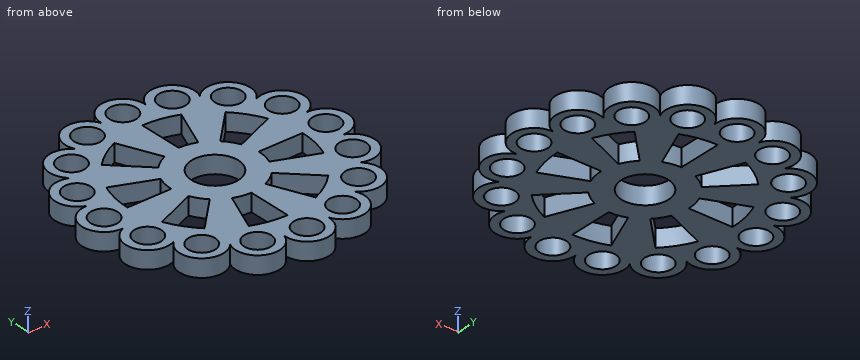
from build123d import *

# Parameters (mm, degrees)
F0_R     = 4.6
F0_R_2   = 8
F1_DEPTH = 6


with BuildPart() as f1:
    # F0 (on Top) → F1 (new body)
    with BuildSketch(Plane.XY):
        with BuildLine():
            ThreePointArc((21.337271, 31.933482), (17.412096, 42.036519), (7.492653, 37.66811))
            ThreePointArc((7.492653, 37.66811), (0, 45.5), (-7.492653, 37.66811))
            ThreePointArc((-7.492653, 37.66811), (-17.412096, 42.036519), (-21.337271, 31.933482))
            ThreePointArc((-21.337271, 31.933482), (-32.173359, 32.173359), (-31.933482, 21.337271))
            ThreePointArc((-31.933482, 21.337271), (-42.036519, 17.412096), (-37.66811, 7.492653))
            ThreePointArc((-37.66811, 7.492653), (-45.5, 0), (-37.66811, -7.492653))
            ThreePointArc((-37.66811, -7.492653), (-42.036519, -17.412096), (-31.933482, -21.337271))
            ThreePointArc((-31.933482, -21.337271), (-32.173359, -32.173359), (-21.337271, -31.933482))
            ThreePointArc((-21.337271, -31.933482), (-17.412096, -42.036519), (-7.492653, -37.66811))
            ThreePointArc((-7.492653, -37.66811), (0, -45.5), (7.492653, -37.66811))
            ThreePointArc((7.492653, -37.66811), (17.412096, -42.036519), (21.337271, -31.933482))
            ThreePointArc((21.337271, -31.933482), (32.173359, -32.173359), (31.933482, -21.337271))
            ThreePointArc((31.933482, -21.337271), (42.036519, -17.412096), (37.66811, -7.492653))
            ThreePointArc((37.66811, -7.492653), (45.5, 0), (37.66811, 7.492653))
            ThreePointArc((37.66811, 7.492653), (42.036519, 17.412096), (31.933482, 21.337271))
            ThreePointArc((31.933482, 21.337271), (32.173359, 32.173359), (21.337271, 31.933482))
        make_face()
        with Locations((-26.870058, -26.870058)):
            Circle(F0_R, mode=Mode.SUBTRACT)
        with Locations((-14.54197, -35.107422)):
            Circle(F0_R, mode=Mode.SUBTRACT)
        with Locations((-35.107422, -14.54197)):
            Circle(F0_R, mode=Mode.SUBTRACT)
        with BuildLine():
            ThreePointArc((-21.213203, -21.213203), (-24.944088, -16.667107), (-27.716386, -11.480503))
            Line((-27.716386, -11.480503), (-13.858193, -5.740251))
            ThreePointArc((-13.858193, -5.740251), (-12.472044, -8.333553), (-10.606602, -10.606602))
            Line((-10.606602, -10.606602), (-21.213203, -21.213203))
        make_face(mode=Mode.SUBTRACT)
        with BuildLine():
            ThreePointArc((0, -30), (-5.85271, -29.423558), (-11.480503, -27.716386))
            Line((-11.480503, -27.716386), (-5.740251, -13.858193))
            ThreePointArc((-5.740251, -13.858193), (-2.926355, -14.711779), (0, -15))
            Line((0, -15), (0, -30))
        make_face(mode=Mode.SUBTRACT)
        with Locations((0, -38)):
            Circle(F0_R, mode=Mode.SUBTRACT)
        with Locations((14.54197, -35.107422)):
            Circle(F0_R, mode=Mode.SUBTRACT)
        with Locations((26.870058, -26.870058)):
            Circle(F0_R, mode=Mode.SUBTRACT)
        with BuildLine():
            ThreePointArc((21.213203, -21.213203), (16.667107, -24.944088), (11.480503, -27.716386))
            Line((11.480503, -27.716386), (5.740251, -13.858193))
            ThreePointArc((5.740251, -13.858193), (8.333553, -12.472044), (10.606602, -10.606602))
            Line((10.606602, -10.606602), (21.213203, -21.213203))
        make_face(mode=Mode.SUBTRACT)
        with BuildLine():
            ThreePointArc((30, 0), (29.423558, -5.85271), (27.716386, -11.480503))
            Line((27.716386, -11.480503), (13.858193, -5.740251))
            ThreePointArc((13.858193, -5.740251), (14.711779, -2.926355), (15, 0))
            Line((15, 0), (30, 0))
        make_face(mode=Mode.SUBTRACT)
        with Locations((35.107422, -14.54197)):
            Circle(F0_R, mode=Mode.SUBTRACT)
        with Locations((-38, 0)):
            Circle(F0_R, mode=Mode.SUBTRACT)
        with Locations((-35.107422, 14.54197)):
            Circle(F0_R, mode=Mode.SUBTRACT)
        with BuildLine():
            ThreePointArc((-30, 0), (-29.423558, 5.85271), (-27.716386, 11.480503))
            Line((-27.716386, 11.480503), (-13.858193, 5.740251))
            ThreePointArc((-13.858193, 5.740251), (-14.711779, 2.926355), (-15, 0))
            Line((-15, 0), (-30, 0))
        make_face(mode=Mode.SUBTRACT)
        with BuildLine():
            ThreePointArc((-21.213203, 21.213203), (-16.667107, 24.944088), (-11.480503, 27.716386))
            Line((-11.480503, 27.716386), (-5.740251, 13.858193))
            ThreePointArc((-5.740251, 13.858193), (-8.333553, 12.472044), (-10.606602, 10.606602))
            Line((-10.606602, 10.606602), (-21.213203, 21.213203))
        make_face(mode=Mode.SUBTRACT)
        with Locations((-26.870058, 26.870058)):
            Circle(F0_R, mode=Mode.SUBTRACT)
        with Locations((-14.54197, 35.107422)):
            Circle(F0_R, mode=Mode.SUBTRACT)
        Circle(F0_R_2, mode=Mode.SUBTRACT)
        with BuildLine():
            ThreePointArc((0, 30), (5.85271, 29.423558), (11.480503, 27.716386))
            Line((11.480503, 27.716386), (5.740251, 13.858193))
            ThreePointArc((5.740251, 13.858193), (2.926355, 14.711779), (0, 15))
            Line((0, 15), (0, 30))
        make_face(mode=Mode.SUBTRACT)
        with BuildLine():
            ThreePointArc((21.213203, 21.213203), (24.944088, 16.667107), (27.716386, 11.480503))
            Line((27.716386, 11.480503), (13.858193, 5.740251))
            ThreePointArc((13.858193, 5.740251), (12.472044, 8.333553), (10.606602, 10.606602))
            Line((10.606602, 10.606602), (21.213203, 21.213203))
        make_face(mode=Mode.SUBTRACT)
        with Locations((38, 0)):
            Circle(F0_R, mode=Mode.SUBTRACT)
        with Locations((35.107422, 14.54197)):
            Circle(F0_R, mode=Mode.SUBTRACT)
        with Locations((0, 38)):
            Circle(F0_R, mode=Mode.SUBTRACT)
        with Locations((14.54197, 35.107422)):
            Circle(F0_R, mode=Mode.SUBTRACT)
        with Locations((26.870058, 26.870058)):
            Circle(F0_R, mode=Mode.SUBTRACT)
    extrude(amount=F1_DEPTH)


solid = f1.part
Verification items for the finished model (mm, model axes). Give positions to 0.01 mm unless a question says otherwise; leave off trailing zeros. Order: outer loops, then holes, each group sorted by start corner. A loop starts at its lowest first (then second) coordinate and runs counter-clockwise, first axis right, second up. Notation, with made-up numbers: (-13.5, 30) -> (24.5, 30) arc R32 cw to (24.5, 63) -> close; hole circle Ø10 at (-12, 1.5). An arc over 180 degrees is marked (long way). Answer as CSV lines item,"result".
Q1. Sectioned sample at C-C on y = -3.5. Record the cut outline in (x, z).
Solutions:
outline,"(-44.63, 0) -> (-40.98, 0) -> (-40.98, 6) -> (-44.63, 6) -> close; (-35.02, 0) -> (-7.19, 0) -> (-7.19, 6) -> (-35.02, 6) -> close; (7.19, 0) -> (14.59, 0) -> (14.59, 6) -> (7.19, 6) -> close; (29.8, 0) -> (35.02, 0) -> (35.02, 6) -> (29.8, 6) -> close; (40.98, 0) -> (44.63, 0) -> (44.63, 6) -> (40.98, 6) -> close"
Q2. Sectioned sample at A-A on y = 24. Record the cut outline in (x, z), plus the area to 3 significant figures.
Solutions:
outline,"(-33.8, 0) -> (-30.46, 0) -> (-30.46, 6) -> (-33.8, 6) -> close; (-23.28, 0) -> (-18, 0) -> (-18, 6) -> (-23.28, 6) -> close; (-9.94, 0) -> (0, 0) -> (0, 6) -> (-9.94, 6) -> close; (9.94, 0) -> (23.28, 0) -> (23.28, 6) -> (9.94, 6) -> close; (30.46, 0) -> (33.8, 0) -> (33.8, 6) -> (30.46, 6) -> close"
area,"211 mm²"
Q3. Scan lines: probe 1 along X at (y, z) = (-9.5, 0.9); probe 2 along X at (y, z) = (-40.5, 0.5); probe 3 along Y at (x, z) = (-36.5, 5.75). Record each from-to range of solid material in increasing order.
Solutions:
probe 1,"x = -40.66 to -22.94, -11.61 to 22.94, 28.46 to 40.66"
probe 2,"x = -19.75 to -9.33, -7.07 to -3.86, 3.86 to 7.07, 9.33 to 19.75"
probe 3,"y = -21.91 to -18.93, -10.16 to -4.35, 4.35 to 10.16, 18.93 to 21.91"
Q4. Depth check by flat-ended pin: pin 1 (10.5 mm diameter, centred on x = 35.11, y = 14.54, fed in from +Z); pin 2 (1 mm diameter, centred on x = 4.5, z = 5, fed in from -Y); pin 3 (2 mm diameter, centred on x = 11.5, z = 5, fed in from +Y); pin 4 (5.5 mm diameter, centred on x = -38, y = 0, fed in from +Z). Enter the tip coordinate at first touch or a pass-through.
Solutions:
pin 1,"stops at z = 6"
pin 2,"stops at y = -44.34"
pin 3,"stops at y = 42.32"
pin 4,"passes through"
Q5. Sectioned sample at B-B on z = 1.3. Count the separate pieces of the cut face and the enclosed holes in it, plus the area to 3 significant figures.
Solutions:
separate pieces,"1"
enclosed holes,"25"
area,"3,680 mm²"
